```python
from build123d import *


with BuildPart() as part:
    # 草图1 → 旋转1 (revolve)
    with BuildSketch(Plane(origin=(0, 0, 0), x_dir=(1, 0, 0), z_dir=(0, 1, 0)), mode=Mode.PRIVATE) as revolve_1_sk:
        Polygon((0, 7), (22.5, 7), (22.5, 11.5), (24.5, 11.5), (24.5, 9), (29, 9), (29, 7.5), (24.5, 7.5), (24.5, 6.5), (24, 6.5), (23, 5.5), (0, 5.5), align=None)
    revolve_1 = revolve(revolve_1_sk.sketch.rotate(Axis((0, 0, 0), (1, 0, 0)), 180), axis=Axis((0, 0, 0), (1, 0, 0)))

    # 镜向1: 旋转1 across plane
    add(revolve_1.mirror(Plane(origin=(0, 0, -5.5), x_dir=(0, 0, 1), z_dir=(1, 0, 0))))


solid = part.part
```
Check sheet for the modelled part. Datum: model origin and axes. Units: mm. A direction names the side the tool comes from. Round coordinates to 2 decimals unless told otherwise and drop trailing zeros. Loops run counter-clockwise (first coordinate to the right, second up) from the corner with the lowest first, then second, coordinate; pieces in that order, holes last. Notation, with made-up numbers: (73.5, 49.5) -> (90.5, 49.5) arc R27 cw to (90.5, 74.5) -> close; hole circle Ø10 at (-22, 1.5). An arc over 180 degrees is marked (long way). Write item = value, one per line. Start each with the question number.
1) Sectioned sample at A-A, the plane x = 7. Record the cut outline in (y, z), plus the area to 3 significant figures.
2) Thickness scan on probe 1 along X at (y, z) = (3.25, 10); probe 2 along Y at (x, z) = (-24.15, 0); probe 3 along X at (y, z) = (-5.5, 6.25). Record the ranges inside material, lowest first.
3) Set-up check for faces 1 (the flat face through (-22.5, 8, 0)), 2 (the flat face through (-24.5, 6, -7)), 3 (the flat face through (24.5, -3, -6)): record each of +Z, -Z, +X, -X, +Y, -Y from which the full face is reachable in a straight line by a thin tool's end or side.
4) Gauge pin test, flat ends, axial feed: pin 1 Ø5 at (x, y) = (0, 6.5) entering from +Z; pin 2 Ø8 at (x, y) = (4.5, -6.5) entering from -Z; pin 3 Ø1 at (x, y) = (-21.5, -4.5) entering from -Z. Record the tip position at first contact, or that the pin passes through.
5) Release check for a two-part mould opening along Z. For faces 4 (the cylindrical face through (-0.315, 2.681, 6.466)), 5 (the flat face through (22.5, 8, 0)), 6 (the cylindrical face through (26.718, -6.324, 4.032)) record: released by +Z, released by -Z, zero draft, split by the parting line, or undercut.
Results are:
q1.outline = circle Ø14 at (0, 0); hole circle Ø11 at (0, 0)
q1.area = 58.9 mm^2
q2.probe_1 = -24.5 to -22.5, 22.5 to 24.5
q2.probe_2 = -11.5 to -6.5, 6.5 to 11.5
q2.probe_3 = -29 to -22.5, 22.5 to 29
q3.face_1 = none
q3.face_2 = -X
q3.face_3 = +X
q4.pin_1 = 5.74
q4.pin_2 = -6.54
q4.pin_3 = -5.74
q5.face_4 = split by the parting line
q5.face_5 = zero draft
q5.face_6 = undercut
